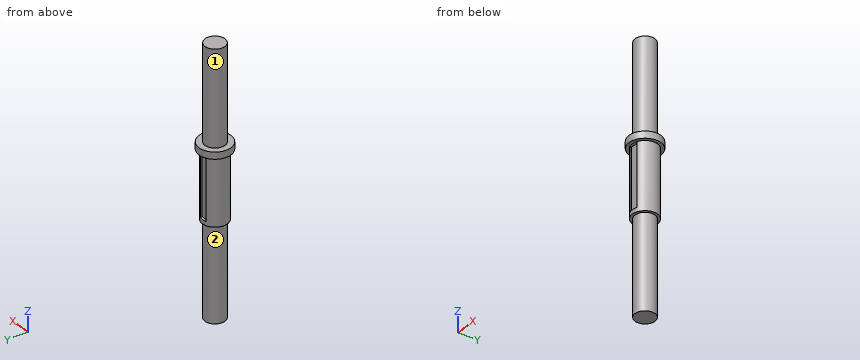
```python
from build123d import *

# Parameters (mm, degrees)
SKETCH1_R           = 6.35
BOSS_EXTRUDE1_DEPTH = 160.3
SKETCH3_OUTSIDE_W   = 46.96
SKETCH3_OUTSIDE_H   = 46.96
SKETCH3_OUTSIDE_R   = 5
CUT_EXTRUDE2_DEPTH  = 120
SKETCH4_OUTSIDE_W   = 46.96
SKETCH4_OUTSIDE_H   = 46.96
SKETCH4_OUTSIDE_R   = 3.96875
CUT_EXTRUDE3_DEPTH  = 37.57
SKETCH5_OUTSIDE_W   = 46.96
SKETCH5_OUTSIDE_H   = 46.96
SKETCH5_OUTSIDE_R   = 3.97
CUT_EXTRUDE4_DEPTH  = 93.36
SKETCH9_W           = 3
SKETCH9_H           = 25
CUT_EXTRUDE6_DEPTH  = 1
SKETCH11_W          = 3.767354336
SKETCH11_H          = 25
CUT_EXTRUDE7_DEPTH  = 1
SKETCH12_R          = 15.914705016
CUT_EXTRUDE8_DEPTH  = 55.98


with BuildPart() as part:
    # Sketch1 → Boss-Extrude1 (new body)
    with BuildSketch(Plane.XY):
        Circle(SKETCH1_R)
    extrude(amount=BOSS_EXTRUDE1_DEPTH)

    # Sketch3 outside → Cut-Extrude2 (cut)
    with BuildSketch(Plane(origin=(0, 0, 0), x_dir=(-1, 0, 0), z_dir=(0, 0, -1))):
        Rectangle(SKETCH3_OUTSIDE_W, SKETCH3_OUTSIDE_H)
        Circle(SKETCH3_OUTSIDE_R, mode=Mode.SUBTRACT)
    extrude(amount=-CUT_EXTRUDE2_DEPTH, mode=Mode.SUBTRACT)

    # Sketch4 outside → Cut-Extrude3 (cut)
    with BuildSketch(Plane.XY.offset(160.3)):
        Rectangle(SKETCH4_OUTSIDE_W, SKETCH4_OUTSIDE_H)
        Circle(SKETCH4_OUTSIDE_R, mode=Mode.SUBTRACT)
    extrude(amount=-CUT_EXTRUDE3_DEPTH, mode=Mode.SUBTRACT)

    # Sketch5 outside → Cut-Extrude4 (cut)
    with BuildSketch(Plane(origin=(0, 0, 0), x_dir=(-1, 0, 0), z_dir=(0, 0, -1))):
        Rectangle(SKETCH5_OUTSIDE_W, SKETCH5_OUTSIDE_H)
        Circle(SKETCH5_OUTSIDE_R, mode=Mode.SUBTRACT)
    extrude(amount=-CUT_EXTRUDE4_DEPTH, mode=Mode.SUBTRACT)

    # Sketch9 → Cut-Extrude6 (cut)
    with BuildSketch(Plane(origin=(0, 5, 0), x_dir=(1, 0, 0), z_dir=(0, 1, 0))):
        with Locations((0, -107.5)):
            Rectangle(SKETCH9_W, SKETCH9_H)
    extrude(amount=-CUT_EXTRUDE6_DEPTH, mode=Mode.SUBTRACT)

    # Sketch11 → Cut-Extrude7 (cut)
    with BuildSketch(Plane(origin=(0, -5, 0), x_dir=(-1, 0, 0), z_dir=(0, -1, 0))):
        with Locations((0, -107.520343873)):
            Rectangle(SKETCH11_W, SKETCH11_H)
    extrude(amount=-CUT_EXTRUDE7_DEPTH, mode=Mode.SUBTRACT)

    # Sketch12 → Cut-Extrude8 (cut)
    with BuildSketch(Plane(origin=(0, 0, 0), x_dir=(-1, 0, 0), z_dir=(0, 0, -1))):
        Circle(SKETCH12_R)
    extrude(amount=-CUT_EXTRUDE8_DEPTH, mode=Mode.SUBTRACT)


solid = part.part
```
Build history of the part. All positions in model axes, mm. Face numbers are marked on the shaded views. A direction names the side the tool comes from. Give positions to 0.01 mm unless a question says otherwise; leave off trailing zeros. Loops run counter-clockwise (first coordinate to the right, second up) from the corner with the lowest first, then second, coordinate; pieces in that order, holes last. Notation, with made-up numbers: (80.25, 68) - (95.25, 68) arc R32 ccw to (95.25, 94) - close; hole circle Ø8 at (-25, 72). An arc over 180 degrees is marked (long way). Use a Markdown table: item, result.
(1) Band-saw the part on A-A (y = 0). Give the cut face in (x, z).
Taken from the geometry:
| item | result |
|---|---|
| outline | (-6.35, 120) - (-5, 120) - (-5, 93.36) - (-3.97, 93.36) - (-3.97, 55.98) - (3.97, 55.98) - (3.97, 93.36) - (5, 93.36) - (5, 120) - (6.35, 120) - (6.35, 122.73) - (3.97, 122.73) - (3.97, 160.3) - (-3.97, 160.3) - (-3.97, 122.73) - (-6.35, 122.73) - close |
(2) Which spindle directions (+Z, -Z, +X, -X, +Y, -Y) get a long thin tool onto all of the face, cutting with end or side? Do the marked faces 1 and 2. Say none if no direction does.
Taken from the geometry:
| item | result |
|---|---|
| face 1 | +Z |
| face 2 | -Z |
(3) Wall check: line 1 along Z through (x, y) = (5, 3.25); line 2 along Z through (x, y) = (-0.75, 4.25); line 3 along Z through (x, y) = (-4.5, -1.75). Give the ranges that are in metal, low to high.
Taken from the geometry:
| item | result |
|---|---|
| line 1 | 120 to 122.73 |
| line 2 | 93.36 to 95, 120 to 122.73 |
| line 3 | 93.36 to 122.73 |
(4) Band-saw the part on C-C (z = 66.5). Give the cut face in (x, y), and give its area (3 significant figures).
Taken from the geometry:
| item | result |
|---|---|
| outline | circle Ø7.94 at (0, 0) |
| area | 49.5 mm2 |
(5) Drop flat-ended pins along their axis: pin 1 Ø6 at (x, z) = (-1, 106) entering from +Y; pin 2 Ø4 at (y, z) = (-2.5, 67.5) entering from -X; pin 3 Ø4 at (x, z) = (1, 103.5) entering from -Y; pin 4 Ø3 at (x, y) = (4, 3) entering from -Z. Give the stop position or say it passes through.
Taken from the geometry:
| item | result |
|---|---|
| pin 1 | y = 4.77 |
| pin 2 | x = -3.94 |
| pin 3 | y = -4.63 |
| pin 4 | z = 55.98 |
